Design review of the part built by this model. Coordinates are the model's own, in mm. A direction names the side the tool comes from. Round coordinates to 2 decimals unless told otherwise and drop trailing zeros. Loops run counter-clockwise (first coordinate to the right, second up) from the corner with the lowest first, then second, coordinate; pieces in that order, holes last. Notation, with made-up numbers: M 24,0 L 67,0 A20 ccw 67,4 Z; hole C 50.25,-30 d11. An arc over 180 degrees is marked long. One line per item, written item: value. Start each with the question number.
Item 1: For line 1 along Y through (x, z) = (20.5, 24.75); line 2 along X through (y, z) = (4.25, 31); line 3 along Z through (x, y) = (8, 5.5), list the stretches that pass through material, from the lowest coordinate up.
Item 2: We need section D-D (y = 4). State how many separate pieces and enclosed holes the cut face has, then the cut area to 3 significant figures.
Item 3: Mouldability with a two-part tool opening along Z and no side actions: class faces 5 (the cylindrical face through (0.9, 7.14, 2.96)), 6 (the cylindrical face through (25.9, 4.06, 25.74)), 7 (the flat face through (6, 4, 32.6)) as released by +Z, released by -Z, zero draft, split by the parting line, or undercut.
Item 4: For faces 1 (the cylindrical face through (21.88, 4.44, 26.47)), 2 (the cylindrical face through (15.14, 4.06, 6.9)), 3 (the cylindrical face through (5.48, 3.39, 29.64)), 4 (the flat face through (40, 4, 26.6)), list the 3-axis set-ups (+Z, -Z, +X, -X, +Y, -Y) from which the entire face can be reached by the end or side of a thin tool; tool diameter is ignored.
Item 5: Clearance check with flat-ended pins moving along their axes: pin 1 (4 mm diameter, centred on x = 6.5, y = 3.5, fed in from +Z); pin 2 (2.5 mm diameter, centred on y = 6, z = 18.5, fed in from -X). State where each tip first meets the part, or that it passes through.
Item 6: We need section C-C (z = 29.5). Write out the cut boundary in (x, y), then the cut area to 3 significant figures.
Item 7: We need section B-B (z = 5). Write out the cut boundary in (x, y).
Item 8: We need section A-A (x = 7). Write out the cut boundary in (y, z).
from build123d import *

# Parameters (mm, degrees)
SKETCH1_W               = 52
SKETCH1_H               = 32.6
BOSS_EXTRUDE1_DEPTH     = 8
SKETCH2_W               = 20.6
SKETCH2_H               = 8
CUT_EXTRUDE1_DEPTH      = 27
SKETCH3_W               = 20.6
SKETCH3_H               = 8
CUT_EXTRUDE2_DEPTH      = 16
SKETCH5_R               = 1.6
CUT_EXTRUDE4_DEPTH      = 62.893133706
FILLET1_R               = 3
FILLET2_R               = 3
SKETCH8_W               = 9
SKETCH8_H               = 8
BOSS_EXTRUDE2_DEPTH     = 3
CUT_EXTRUDE5_DEPTH      = 4
CUT_EXTRUDE5_DEPTH_BACK = 15
SKETCH6_R               = 1.45
FILLET3_R               = 4


with BuildPart() as part:
    # Sketch1 → Boss-Extrude1 (new body)
    with BuildSketch(Plane(origin=(0, 0, 0), x_dir=(1, 0, 0), z_dir=(0, 1, 0))):
        with Locations((26, -16.3)):
            Rectangle(SKETCH1_W, SKETCH1_H)
    extrude(amount=BOSS_EXTRUDE1_DEPTH)

    # Sketch2 → Cut-Extrude1 (cut)
    with BuildSketch(Plane(origin=(52, 0, 0), x_dir=(0, 0, -1), z_dir=(1, 0, 0))):
        with Locations((-16.3, 4)):
            Rectangle(SKETCH2_W, SKETCH2_H)
    extrude(amount=-CUT_EXTRUDE1_DEPTH, mode=Mode.SUBTRACT)

    # Sketch3 → Cut-Extrude2 (cut)
    with BuildSketch(Plane.ZY):
        with Locations((16.3, 4)):
            Rectangle(SKETCH3_W, SKETCH3_H)
    extrude(amount=-CUT_EXTRUDE2_DEPTH, mode=Mode.SUBTRACT)

    # Sketch5 → Cut-Extrude4 (cut, through all)
    with BuildSketch(Plane.XY.offset(32.6)):
        with Locations((4, 4)):
            Circle(SKETCH5_R)
        with Locations((48, 4)):
            Circle(SKETCH5_R)
    extrude(amount=-CUT_EXTRUDE4_DEPTH, mode=Mode.SUBTRACT)

    # Fillet1
    fillet1_edges = [part.edges().sort_by_distance(p)[0] for p in [
        (52, 8, 29.6),
        (52, 0, 3),
        (52, 8, 3),
        (0, 0, 29.6),
        (0, 8, 29.6),
        (0, 8, 3),
        (52, 0, 29.6),
        (0, 0, 3),
    ]]
    fillet(fillet1_edges, radius=FILLET1_R)

    # Fillet2
    fillet2_edges = [part.edges().sort_by_distance(p)[0] for p in [
        (25, 4, 26.6),
        (25, 4, 6),
        (16, 4, 6),
        (16, 4, 26.6),
    ]]
    fillet(fillet2_edges, radius=FILLET2_R)

    # Sketch8 → Boss-Extrude2 (add)
    with BuildSketch(Plane.XY.offset(32.6)):
        with Locations((20.5, 4)):
            Rectangle(SKETCH8_W, SKETCH8_H)
    extrude(amount=BOSS_EXTRUDE2_DEPTH)

    # Sketch6 → Cut-Extrude5 (cut, two sides: drawn at the far end of the back side and taken through both)
    with BuildSketch(Plane.XY.offset(32.6).offset(-CUT_EXTRUDE5_DEPTH_BACK)):
        with Locations((20.5, 4)):
            Circle(SKETCH6_R)
    extrude(amount=CUT_EXTRUDE5_DEPTH + CUT_EXTRUDE5_DEPTH_BACK, mode=Mode.SUBTRACT)

    # Fillet3
    # the kernel refuses this fillet: 4 mm, written as the material it adds along each edge
    with BuildSketch(Plane(origin=(25, 8, 32.6), x_dir=(0, 0, 1), z_dir=(0, -1, 0))) as fillet3_piece_1:
        with BuildLine():
            CenterArc((4, -3.872983346), FILLET3_R, 104.477512186, 75.522487814)
            Line((0, -3.872983346), (-0.08, -3.872983346))
            Line((-0.08, -3.872983346), (-0.08, 0))
            Line((-0.08, 0), (0, 0.08))
            ThreePointArc((0, 0.08), (1.5, 0.08), (2.98, 0.077459667))
            Line((2.98, 0.077459667), (3, 0))
        make_face()
    extrude(amount=8)
    with BuildSketch(Plane(origin=(16, 0, 32.6), x_dir=(-1, 0, 0), z_dir=(0, 1, 0))) as fillet3_piece_2:
        with BuildLine():
            CenterArc((3.872983346, 4), FILLET3_R, 194.477512186, 75.522487814)
            Line((0, 3), (-0.077459667, 2.98))
            ThreePointArc((-0.077459667, 2.98), (-0.08, 1.5), (-0.08, 0))
            Line((-0.08, 0), (0, -0.08))
            Line((0, -0.08), (3.872983346, -0.08))
            Line((3.872983346, -0.08), (3.872983346, 0))
        make_face()
    extrude(amount=8)


solid = part.part
A:
1. line 1: 0 to 2.55, 5.45 to 8
1. line 2: 0 to 2.42, 5.58 to 19.07, 21.93 to 46.42, 49.58 to 52
1. line 3: 0 to 6, 26.6 to 32.6
2. separate pieces: 5
2. enclosed holes: 0
2. area: 721 mm2
3. face 5: zero draft
3. face 6: undercut
3. face 7: released by +Z
4. face 1: +Z
4. face 2: -X, +Y, -Y
4. face 3: +Z, -Z
4. face 4: +X, +Y, -Y
5. pin 1: z = 32.6
5. pin 2: x = 16
6. outline: M 0,3 A3 ccw 3,0 L 49,0 A3 ccw 52,3 L 52,5 A3 ccw 49,8 L 3,8 A3 ccw 0,5 Z; hole C 4,4 d3.2; hole C 20.5,4 d2.9; hole C 48,4 d3.2
6. area: 386 mm2
7. outline: M 0,3 A3 ccw 3,0 L 49,0 A3 ccw 52,3 L 52,5 A3 ccw 49,8 L 3,8 A3 ccw 0,5 Z; hole C 4,4 d3.2; hole C 48,4 d3.2
8. outline: M 0,0 L 8,0 L 8,6 L 0,6 Z; M 0,26.6 L 8,26.6 L 8,32.6 L 0,32.6 Z
